Geometry check sheet. Reference: the model listing, model coordinates, mm. A direction names the side the tool comes from. Round coordinates to 2 decimals unless told otherwise and drop trailing zeros. Order: outer loops, then holes, each group sorted by start corner. A loop starts at its lowest first (then second) coordinate and runs counter-clockwise, first axis right, second up. Notation, with made-up numbers: (36, -20) -> (68, -20) arc R21 cw to (68, -2) -> close; hole circle Ø1 at (-28.5, 41). An arc over 180 degrees is marked (long way). Answer as a JSON object with one key per item and string values. Group by question number.
from build123d import *

# Parameters (mm, degrees)
SKETCH_2_W             = 64.02174429
SKETCH_2_H             = 9.248919907
CUT_EXTRUDE_1_DEPTH    = 49
HOLE_WIZARD_M4_2_D     = 3.3
HOLE_WIZARD_M4_2_DEPTH = 5.5
HOLE_WIZARD_M4_2_TIP   = 0.991420021
HOLE_WIZARD_M6_2_D     = 5
HOLE_WIZARD_M6_2_DEPTH = 5.5
HOLE_WIZARD_M6_2_TIP   = 1.502151548


with BuildPart() as part:
    # 草图1 → 旋转1 (revolve)
    with BuildSketch(Plane(origin=(0, 0, 0), x_dir=(1, 0, 0), z_dir=(0, 1, 0)), mode=Mode.PRIVATE) as revolve_1_sk:
        Polygon((29.5, 7.5), (29.5, -7.5), (20.5, -7.5), (20.5, -3), (21.1, -3), (21.1, -2), (19, -2), (19, 2), (21.1, 2), (21.1, 3), (20.5, 3), (20.5, 7.5), align=None)
    revolve(revolve_1_sk.sketch.rotate(Axis((0, 0, -31.9390681), (0, 0, 1)), 180), axis=Axis((0, 0, -31.9390681), (0, 0, 1)))  # turned: the seam where the file's is

    # 草图2 → 切除-拉伸1 (cut)
    with BuildSketch(Plane.XY.offset(7.5)):
        with Locations((-1.141100508, 33.324459954)):
            Rectangle(SKETCH_2_W, SKETCH_2_H)
        with Locations((-1.141100508, -33.324459954)):
            Rectangle(SKETCH_2_W, SKETCH_2_H)
    extrude(amount=-CUT_EXTRUDE_1_DEPTH, mode=Mode.SUBTRACT)

    # M4 螺纹孔2
    with Locations(Plane(origin=(0, 28.7, 0), x_dir=(1, 0, 0), z_dir=(0, 1, 0))):
        with Locations((0, 0)):
            Hole(HOLE_WIZARD_M4_2_D / 2, depth=HOLE_WIZARD_M4_2_DEPTH)
            with Locations((0, 0, -(HOLE_WIZARD_M4_2_DEPTH + HOLE_WIZARD_M4_2_TIP / 2))):  # 118° drill point
                Cone(0, HOLE_WIZARD_M4_2_D / 2, HOLE_WIZARD_M4_2_TIP, mode=Mode.SUBTRACT)

    # M6 螺纹孔2
    with Locations(Plane(origin=(0, -28.7, 0), x_dir=(-1, 0, 0), z_dir=(0, -1, 0))):
        with Locations((0, 0)):
            Hole(HOLE_WIZARD_M6_2_D / 2, depth=HOLE_WIZARD_M6_2_DEPTH)
            with Locations((0, 0, -(HOLE_WIZARD_M6_2_DEPTH + HOLE_WIZARD_M6_2_TIP / 2))):  # 118° drill point
                Cone(0, HOLE_WIZARD_M6_2_D / 2, HOLE_WIZARD_M6_2_TIP, mode=Mode.SUBTRACT)


solid = part.part
Item 1: Set-up check for faces 1 (the cylindrical face through (-0.54, -25.91, 2.44)), 2 (the flat face through (-19, -3, -2)), 3 (the cylindrical face through (-18.937, 7.852, -5.281)): record each of +Z, -Z, +X, -X, +Y, -Y from which the full face is reachable in a straight line by a thin tool's end or side.
Item 2: Thickness scan on L1, parallel to Y at x = 0, z = 5.3; L2, parallel to Z at x = 0, y = -25; L3, parallel to X at y = -19, z = -7. Record the ranges inside material, lowest first.
Item 3: Sectioned sample at A-A, the plane y = 0. Enter the section's corners in (x, z), then the cut area to 3 significant figures.
Item 4: Depth check by flat-ended pin: pin 1 Ø2 at (x, z) = (0, 0) entering from +Y; pin 2 Ø3 at (y, z) = (-13.5, 4) entering from -X; pin 3 Ø6 at (y, z) = (18, -1.5) entering from -X; pin 4 Ø21 at (x, y) = (3, 2) entering from +Z. Enter the tip coordinate at first touch or a pass-through.
Item 5: Mould release check, pull along Z, two halves, no side actions. Record for faces 4 (the cylindrical face through (29.495, -0.552, 0.105)), 5 (the flat face through (7, -20, 7.5)), 6 (the flat face through (-3.22, -20.42, 3)), 7 (the cylindrical face through (-20.126, -6.338, 2.493)): pulls with the +Z half, pulls with the -Z half, needs draft (parallel to the pull), parting line crosses it, or undercut.
Item 6: Sectioned sample at B-B, the plane z = 4. Enter the section's corners in (x, y).
Item 7: Sectioned sample at C-C, the plane y = -9. Enter the section's corners in (x, z), then the cut area to 3 significant figures.
Result:
{
 "1": {"face 1": "-Y", "face 2": "none", "face 3": "-Z"},
 "2": {"L1": "y = -28.7 to -20.5, 20.5 to 28.7", "L2": "z = -7.5 to -2.5, 2.5 to 7.5", "L3": "x = -22.57 to -7.7, 7.7 to 22.57"},
 "3": {"outline": "(-29.5, -7.5) -> (-20.5, -7.5) -> (-20.5, -3) -> (-21.1, -3) -> (-21.1, -2) -> (-19, -2) -> (-19, 2) -> (-21.1, 2) -> (-21.1, 3) -> (-20.5, 3) -> (-20.5, 7.5) -> (-29.5, 7.5) -> close; (19, -2) -> (21.1, -2) -> (21.1, -3) -> (20.5, -3) -> (20.5, -7.5) -> (29.5, -7.5) -> (29.5, 7.5) -> (20.5, 7.5) -> (20.5, 3) -> (21.1, 3) -> (21.1, 2) -> (19, 2) -> close", "area": "280 mm2"},
 "4": {"pin 1": "stops at y = 22.81", "pin 2": "stops at x = -26.95", "pin 3": "stops at x = -25.4", "pin 4": "passes through"},
 "5": {"face 4": "needs draft", "face 5": "pulls with the +Z half", "face 6": "undercut", "face 7": "undercut"},
 "6": {"outline": "(-6.82, -28.7) -> (6.82, -28.7) arc R29.5 ccw to (6.82, 28.7) -> (-6.82, 28.7) arc R29.5 ccw to start; hole circle Ø41 at (0, 0)"},
 "7": {"outline": "(-28.09, -7.5) -> (-18.42, -7.5) -> (-18.42, -3) -> (-19.08, -3) -> (-19.08, -2) -> (-16.73, -2) -> (-16.73, 2) -> (-19.08, 2) -> (-19.08, 3) -> (-18.42, 3) -> (-18.42, 7.5) -> (-28.09, 7.5) -> close; (16.73, -2) -> (19.08, -2) -> (19.08, -3) -> (18.42, -3) -> (18.42, -7.5) -> (28.09, -7.5) -> (28.09, 7.5) -> (18.42, 7.5) -> (18.42, 3) -> (19.08, 3) -> (19.08, 2) -> (16.73, 2) -> close", "area": "301 mm2"}
}
